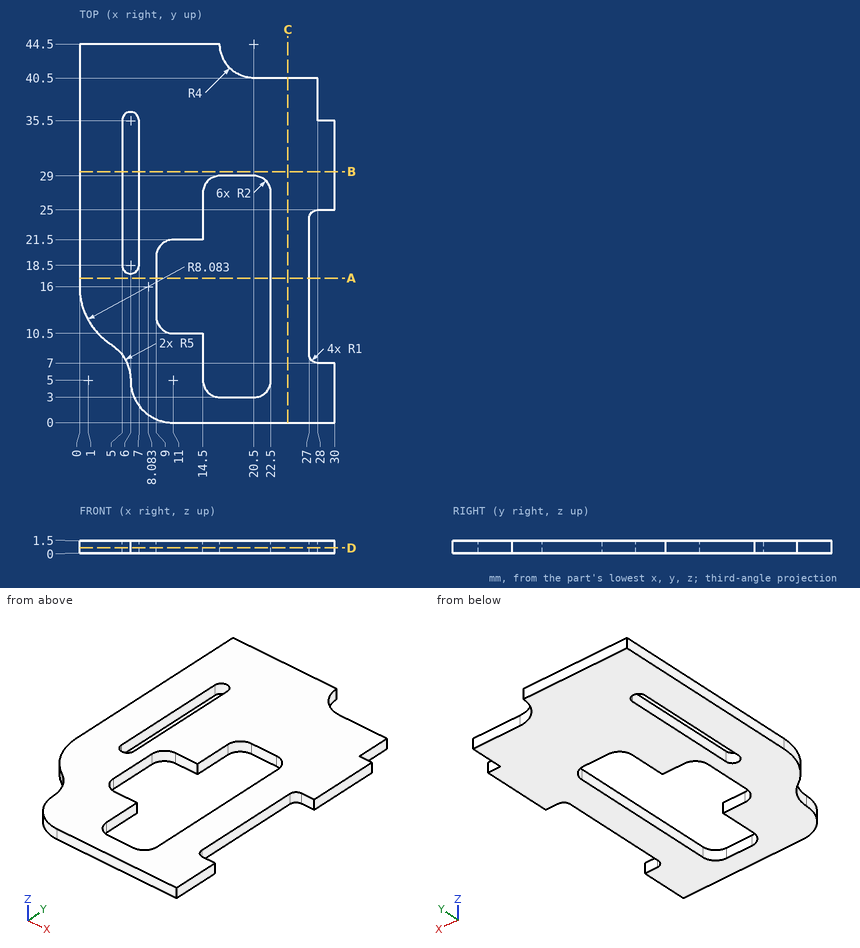
Input: dimensioned drawing with shaded views. Units: mm. Origin: part minimum x, y, z. Coordinates: 2 decimals unless noted, no trailing zeros. Write each loop counter-clockwise with the first axis right and the second up, starting at its lowest first coordinate (ties: lowest second). Pieces come first, ordered by that corner, then holes. Notation, with made-up numbers: M 67,41.25 L 96,41.25 A5 ccw 96,49.25 Z; hole C 35,-33.5 d4. An arc over 180 degrees is marked long. Use a Markdown table: item, result.
1) Section B-B, the plane y = 29.5. Output: boundary loops of the cut face in (x, z), then the cut area to 3 significant figures.
Conclusion:
| item | result |
|---|---|
| outline | M 0,0 L 5,0 L 5,1.5 L 0,1.5 Z; M 7,0 L 30,0 L 30,1.5 L 7,1.5 Z |
| area | 42.0 mm^2 |
2) Section A-A, the plane y = 17. Output: boundary loops of the cut face in (x, z).
Conclusion:
| item | result |
|---|---|
| outline | M 0,0 L 9,0 L 9,1.5 L 0,1.5 Z; M 22.5,0 L 27,0 L 27,1.5 L 22.5,1.5 Z |
3) First-contact query: pin 1 Ø0.8 at (x, z) = (24, 1) entering from +Y; pin 2 Ø0.8 at (y, z) = (23.5, 0.5) entering from +X. Flat tips, straight axial feed; report the tip coordinate or a pass-through.
Conclusion:
| item | result |
|---|---|
| pin 1 | stops at y = 40.5 |
| pin 2 | stops at x = 27 |
4) Section D-D, the plane z = 0.65. Give the number of separate pieces and of enclosed holes in the cut face, then the cut area to 3 significant figures.
Conclusion:
| item | result |
|---|---|
| separate pieces | 1 |
| enclosed holes | 2 |
| area | 855 mm^2 |
5) Section C-C, the plane x = 24.5. Output: boundary loops of the cut face in (y, z).
Conclusion:
| item | result |
|---|---|
| outline | M 0,0 L 40.5,0 L 40.5,1.5 L 0,1.5 Z |
6) Ray query, L1, parallel to X at y = 18.5, z = 0.2; L2, parallel to X at y = 16.5, z = 0.15; L3, parallel to X at y = 28, z = 0.35. Return the intervals inside material, ascending.
Conclusion:
| item | result |
|---|---|
| L1 | x = 0 to 5, 7 to 9, 22.5 to 27 |
| L2 | x = 0 to 9, 22.5 to 27 |
| L3 | x = 0 to 5, 7 to 14.77, 22.23 to 30 |
